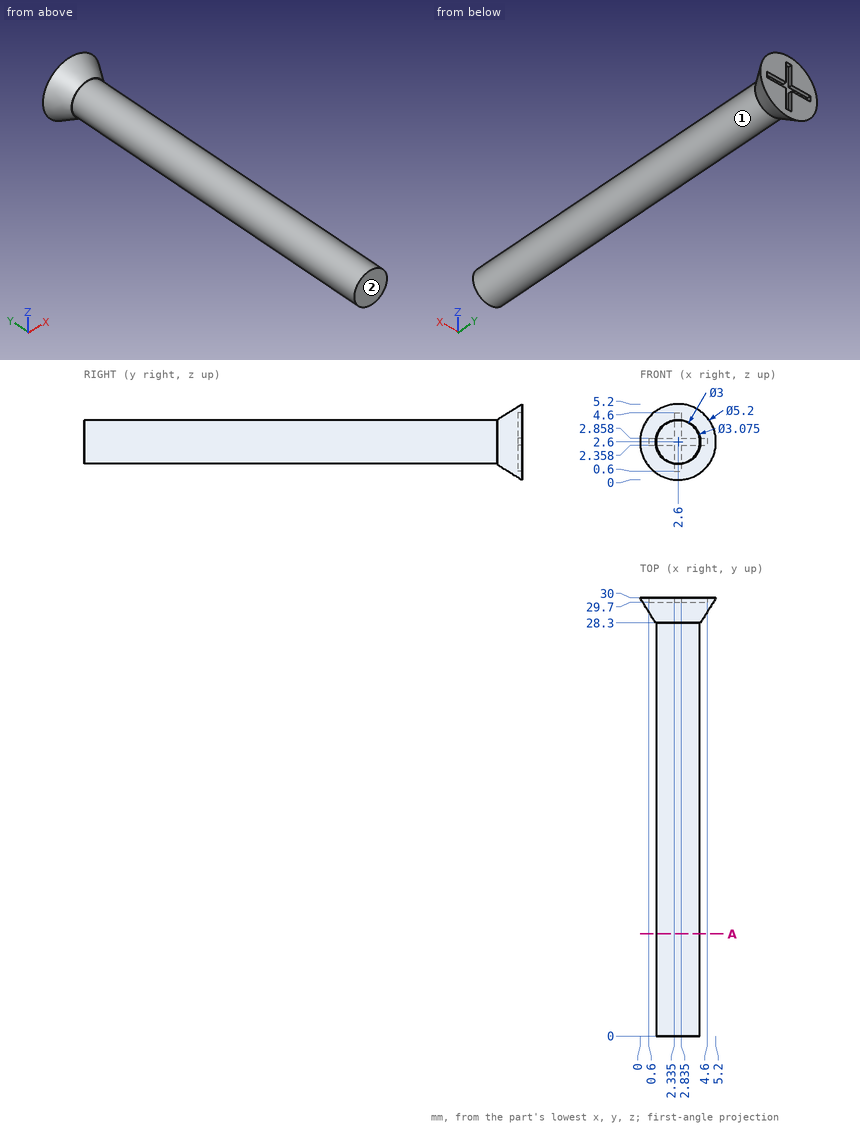
Job drawing, mm, ordinate dimensions from the low corner. One solid piece. A direction names the side the tool comes from. Coordinates: 2 decimals unless noted, no trailing zeros. Order: outer loops, then holes, each group sorted by start corner. A loop starts at its lowest first (then second) coordinate and runs counter-clockwise, first axis right, second up. Notation, with made-up numbers: (65, 39) -> (71, 39) arc R5 ccw to (71, 44) -> close; hole circle Ø5 at (7, 48). An arc over 180 degrees is marked (long way). Return JSON: item names as keys, results as strings. Group by question number.
Item 1: Wall check: line 1 along Y through (x, z) = (2.5, 1.55); line 2 along Z through (x, y) = (2.55, 23). Give the ranges that are in metal, low to high. Write a range as [from, to].
Item 2: Tool access for the marked faces 1 and 2: list every direction of +Z, -Z, +X, -X, +Y, -Y with a clear straight run to the whole face (end or side of a thin tool).
Item 3: Flat gauge pins, fed straight in: P1, Ø1.5, axis at x = 2.5, y = 15, coming from the -Z side; P2, Ø2.5, axis at x = 2.5, z = 2, coming from the -Y side; P3, Ø3, axis at y = 5, z = 1, coming from the +X side; P4, Ø1.5, axis at x = 4.5, y = 24, coming from the +Z side (1 decimal). Where does each tip first touch, or does it go through?
Item 4: Saw through at A-A on y = 7. Write the cut outline in (x, z).
Values found:
{
 "1": {"line 1": "y = [0, 29.7]", "line 2": "z = [1.1, 4.1]"},
 "2": {"face 1": "-Y", "face 2": "+Z, -Z, +X, -X, -Y"},
 "3": {"P1": "stops at z = 1.1", "P2": "stops at y = 0", "P3": "stops at x = 4.1", "P4": "stops at z = 3.6"},
 "4": {"outline": "circle Ø3 at (2.6, 2.6)"}
}
